```python
from build123d import *

# Parameters (mm, degrees)
F1_DEPTH = 5
F2_W     = 3
F2_H     = 5
F3_DEPTH = 6


with BuildPart() as f1:
    # F0 (on Top) → F1 (new body)
    with BuildSketch(Plane.XY):
        with BuildLine():
            ThreePointArc((9.997487, 0), (9.66119, 3.000141), (10, 6))
            Line((10, 6), (0, 6))
            Line((0, 6), (0, 0))
            Line((0, 0), (9.997487, 0))
        make_face()
    extrude(amount=F1_DEPTH)

    # F2 (on face) → F3 (join)
    with BuildSketch(Plane.XZ):
        with Locations((1.5, -2.5)):
            Rectangle(F2_W, F2_H)
    extrude(amount=-F3_DEPTH)


solid = f1.part
```
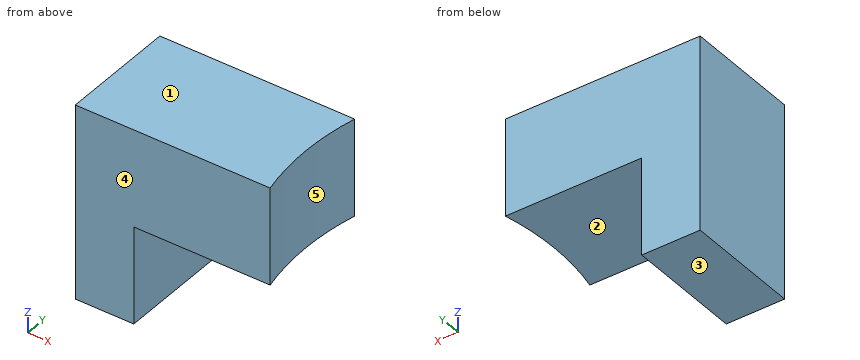
Build history of the part. All positions in model axes, mm. Face numbers are marked on the shaded views. A direction names the side the tool comes from. Round coordinates to 2 decimals unless told otherwise and drop trailing zeros. Order: outer loops, then holes, each group sorted by start corner. A loop starts at its lowest first (then second) coordinate and runs counter-clockwise, first axis right, second up. Notation, with made-up numbers: (-31.5, -15.75) -> (18.5, -15.75) arc R22 cw to (18.5, 22.25) -> close; hole circle Ø10 at (-14.5, 32). An arc over 180 degrees is marked (long way). Answer in a Markdown table with one row per item.
1) Band-saw the part on A-A on z = -2.75. Give the cut face in (x, y).
Values:
| item | result |
|---|---|
| outline | (0, 0) -> (3, 0) -> (3, 6) -> (0, 6) -> close |
2) Mould opens along Y. For the marked faces 3, 4 and 5 say: released by +Y, released by -Y, zero draft, split by the parting line, or undercut.
Values:
| item | result |
|---|---|
| face 3 | zero draft |
| face 4 | released by -Y |
| face 5 | undercut |
3) Band-saw the part on B-B on y = 5.5. Give the cut face in (x, z).
Values:
| item | result |
|---|---|
| outline | (0, -5) -> (3, -5) -> (3, 0) -> (9.9, 0) -> (9.9, 5) -> (0, 5) -> close |
4) Band-saw the part on C-C on x = 6. Give the cut face in (y, z).
Values:
| item | result |
|---|---|
| outline | (0, 0) -> (6, 0) -> (6, 5) -> (0, 5) -> close |
5) Pin check, flat tips, straight feed: P1, Ø3, axis at x = 6.5, y = 2, coming from the -Z side; P2, Ø1, axis at y = 3, z = 1.5, coming from the +X side. Stop position of each tip, or through.
Values:
| item | result |
|---|---|
| P1 | z = 0 |
| P2 | x = 9.67 |
6) Which spindle directions (+Z, -Z, +X, -X, +Y, -Y) get a long thin tool onto all of the face, cutting with end or side? Do the marked faces 1 and 2. Say none if no direction does.
Values:
| item | result |
|---|---|
| face 1 | +Z, +X, -X, +Y, -Y |
| face 2 | -Z, +X, +Y, -Y |
7) Wall check: L1, parallel to Z at x = 8.25, y = 1; L2, parallel to X at y = 5.5, z = -2.25; L3, parallel to X at y = 0.5, z = 2.25. Give the ranges that are in metal, low to high.
Values:
| item | result |
|---|---|
| L1 | 0 to 5 |
| L2 | 0 to 3 |
| L3 | 0 to 9.89 |
8) Band-saw the part on D-D on y = 3.25. Give the cut face in (x, z), and give its area (3 significant figures).
Values:
| item | result |
|---|---|
| outline | (0, -5) -> (3, -5) -> (3, 0) -> (9.66, 0) -> (9.66, 5) -> (0, 5) -> close |
| area | 63.3 mm2 |
